Design review of the part shown in the three views and the two pictorial views. Dimensions are in mm from the part's minimum x, y and z. A direction names the side the tool comes from. Coordinates: 2 decimals unless noted, no trailing zeros. Loops run counter-clockwise (first coordinate to the right, second up) from the corner with the lowest first, then second, coordinate; pieces in that order, holes last. Notation, with made-up numbers: (-40, 16.5) -> (-12, 16.5) arc R16 ccw to (-12, 37.5) -> close; hole circle Ø5 at (-20.75, -21.5). An arc over 180 degrees is marked (long way). Use a Markdown table: item, result. Add a question column.
Q1. For the marked faces 1, 2 and 3, list the 3-axis set-ups (+Z, -Z, +X, -X, +Y, -Y) from which the entire face can be reached by the end or side of a thin tool; tool diameter is ignored.
Q2. Take a section at A-A on y = 20. Write out the cut boundary in (x, z), plus the area to 3 significant figures.
Q3. For probe 1 along Z at (x, y) = (25.5, 7); probe 2 along X at (y, z) = (9, 260.5); probe 3 along X at (y, z) = (12.5, 51), list the stretches that pass through material, from the lowest coordinate up.
Q4. Take a section at C-C on z = 127. Write out the cut boundary in (x, y), plus the area to 3 significant figures.
Q5. Clearance check with flat-ended pins moving along their axes: pin 1 Ø1 at (x, y) = (21, 35) entering from -Z; pin 2 Ø6 at (y, z) = (17, 112) entering from +X; pin 3 Ø2 at (x, y) = (8, 13.5) entering from +Z; pin 4 Ø6 at (y, z) = (23.5, 219.5) entering from -X. State where each tip first meets the part, or that it passes through.
Q6. Take a section at D-D on z = 34.5. Write out the cut boundary in (x, y), plus the area to 3 significant figures.
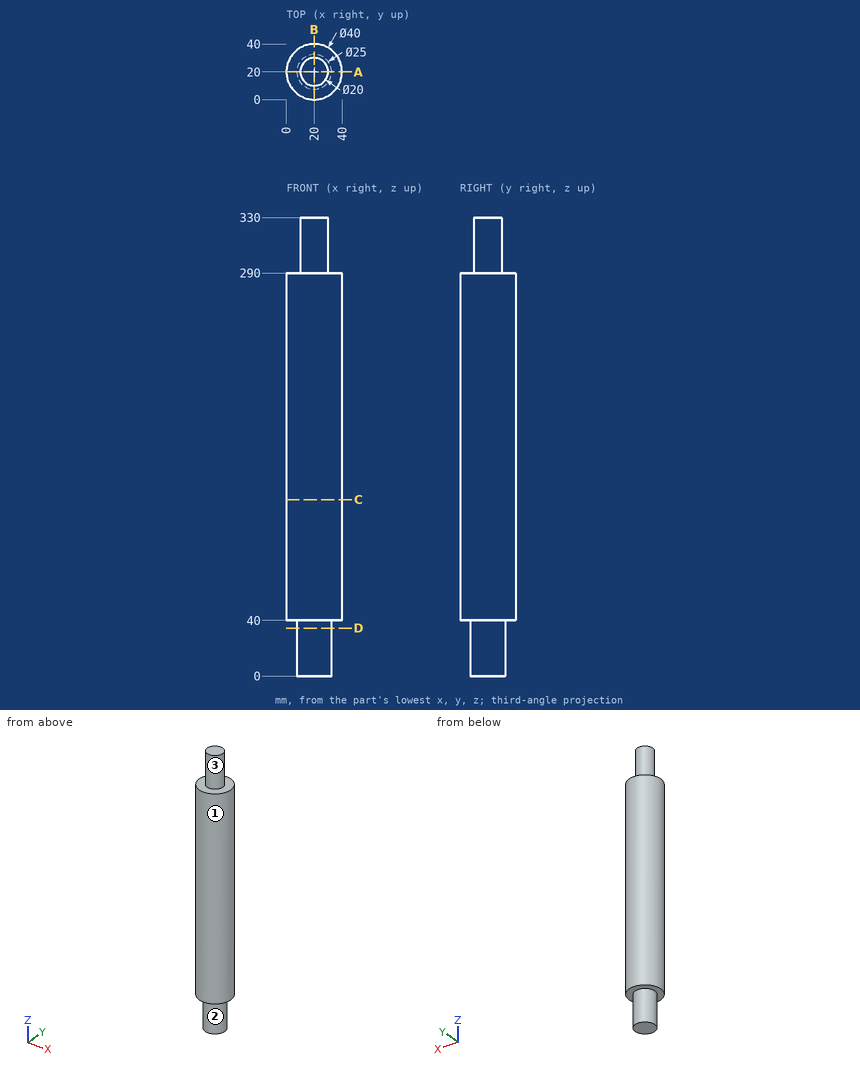
Answer list:
| question | item | result |
|---|---|---|
| 1 | face 1 | +Z, -Z |
| 1 | face 2 | -Z |
| 1 | face 3 | +Z |
| 2 | outline | (0, 40) -> (7.5, 40) -> (7.5, 0) -> (32.5, 0) -> (32.5, 40) -> (40, 40) -> (40, 290) -> (30, 290) -> (30, 330) -> (10, 330) -> (10, 290) -> (0, 290) -> close |
| 2 | area | 11,800 mm² |
| 3 | probe 1 | 40 to 290 |
| 3 | probe 2 | 3.3 to 36.7 |
| 3 | probe 3 | 1.46 to 38.54 |
| 4 | outline | circle Ø40 at (20, 20) |
| 4 | area | 1,260 mm² |
| 5 | pin 1 | z = 40 |
| 5 | pin 2 | x = 40 |
| 5 | pin 3 | z = 290 |
| 5 | pin 4 | x = 0.01 |
| 6 | outline | circle Ø25 at (20, 20) |
| 6 | area | 491 mm² |
